Check sheet for the modelled part. Datum: model origin and axes. Units: mm. A direction names the side the tool comes from. Coordinates: 2 decimals unless noted, no trailing zeros. Write each loop counter-clockwise with the first axis right and the second up, starting at its lowest first coordinate (ties: lowest second). Pieces come first, ordered by that corner, then holes. Notation, with made-up numbers: M 55,14 L 105,14 A14 cw 105,28 Z; hole C 42,70 d4. An arc over 180 degrees is marked long. Answer as CSV lines item,"result".
Autodesk Inventor part; units mm, degrees
ref_plane "YZ Plane" through (0, 0, 0) normal (1, 0, 0) x (0, 1, 0)
ref_plane "XZ Plane" through (0, 0, 0) normal (0, 1, 0) x (-1, 0, 0)
ref_plane "XY Plane" through (0, 0, 0) normal (0, 0, 1) x (1, 0, 0)
sketch "Sketch1" plane through (0, 0, 0) normal (0, 0, 1) x (1, 0, 0)
  line L0 (0, 0) -> (25.4, 0)
  line L1 (25.4, 0) -> (25.4, 25.4)
  line L2 (25.4, 25.4) -> (0, 25.4)
  line L3 (0, 25.4) -> (0, 0)
  line L4 (3.175, 22.225) -> (22.225, 22.225)
  line L5 (22.225, 22.225) -> (22.225, 3.175)
  line L6 (22.225, 3.175) -> (3.175, 3.175)
  line L7 (3.175, 3.175) -> (3.175, 22.225)
  dimension "d0" = 25.4
  dimension "d1" = 25.4
  dimension "d2" = 3.175
extrude "Extrusion1" add sketch "Sketch1" against normal blind 412.75
sketch "Sketch2" plane through (0, 25.4, 0) normal (0, 1, 0) x (1, 0, 0)
  line L0 (25.4, 412.75) -> (0, 412.75)
  line L1 (25.4, 0) -> (0, 0)
  point P0 (12.7, 87.3125)
  point P1 (12.7, 325.4375)
  dimension "d5" = 87.3125
  dimension "d6" = 87.3125
hole "Hole1" at (12.7, 25.4, -87.3125) at (12.7, 25.4, -325.4375) direction (0, -1, 0) diameter 12.7 depth 25.4 tip angle 118
properties part number "16.25inch tube"
1) Section check B-B, the plane y = 13. Record the boundary of the cut face in (x, z) (3 decimals), plus the area to 3 significant figures.
Answer key:
outline,"M 0,-412.75 L 3.175,-412.75 L 3.175,0 L 0,0 Z; M 22.225,-412.75 L 25.4,-412.75 L 25.4,0 L 22.225,0 Z"
area,"2,620 mm2"
2) Section check C-C, the plane z = -342. Record the boundary of the cut face in (x, y) (3 decimals).
Answer key:
outline,"M 0,0 L 25.4,0 L 25.4,25.4 L 0,25.4 Z; hole M 3.175,3.175 L 22.225,3.175 L 22.225,22.225 L 3.175,22.225 Z"
3) Tool access check on faces 1 (the face through (13, 22.225, -203)), 2 (the face through (13, 25.4, -203)). Record the directions out of +Z, -Z, +X, -X, +Y, -Y that give a thin tool (end or side, any length) a straight path to the whole face; none if there is none.
Answer key:
face 1,"+Z, -Z"
face 2,"+Z, -Z, +X, -X, +Y"
4) Mould release check, pull along X, two halves, no side actions. Record for faces 3 (the face through (13, 3.175, -203)), 4 (the face through (0, 13, -203)), 5 (the face through (13, 0, -203)): pulls with the +X half, pulls with the -X half, needs draft (parallel to the pull), parting line crosses it, or undercut.
Answer key:
face 3,"undercut"
face 4,"pulls with the -X half"
face 5,"needs draft"
5) Section check A-A, the plane x = 12.7. Give the number of separate pieces and of enclosed holes in the cut face, plus the area to 3 significant figures.
Answer key:
separate pieces,"6"
enclosed holes,"0"
area,"2,460 mm2"
6) Thickness scan on line 1 along Z through (x, y) = (12.7, 23.25); line 2 along X through (y, z) = (7.75, -319.5) (3 decimals). Record the ranges inside material, lowest first.
Answer key:
line 1,"z = -412.75 to -331.79, -319.09 to -93.66, -80.96 to 0"
line 2,"x = 0 to 3.175, 22.225 to 25.4"
